Verification items for the finished model (mm, model axes). Coordinates: 2 decimals unless noted, no trailing zeros. Write each loop counter-clockwise with the first axis right and the second up, starting at its lowest first coordinate (ties: lowest second). Pieces come first, ordered by that corner, then holes. Notation, with made-up numbers: (53, -37.5) -> (61, -37.5) arc R15 cw to (61, -22.5) -> close; hole circle Ø7 at (14.5, -22.75). An arc over 180 degrees is marked (long way). Write item = value, one per line. Start each with the question number.
(1) Material ranges on probe 1 along X at (y, z) = (2.2, -17.96); probe 2 along X at (y, z) = (3.8, -18); probe 3 along Z at (x, y) = (3.5, 1.7), recorded low to high. Write a range as [from, to].
(2) Section check C-C (x = 9.5). Record the cut outline in (y, z), plus the area to 3 significant figures.
(3) Section check B-B (y = 3.15). Record the cut outline in (x, z), plus the area to 3 significant figures.
(4) Section check A-A (x = 24.56). Record the cut outline in (y, z).
(5) Gauge pin test, flat end, axial feed: pin 1 Ø0.6 at (x, y) = (13, 3.5) entering from +Z. Record the tip position at first contact, or that the pin passes through.
```python
from build123d import *

# Parameters (mm, degrees)
SKETCH1_W           = 27.1
SKETCH1_H           = 20.5
BOSS_EXTRUDE1_DEPTH = 4
SKETCH3_R           = 1.27
CUT_EXTRUDE1_DEPTH  = 35.214909031
SKETCH2_W           = 10.16
SKETCH2_H           = 1.27
SKETCH2_W_2         = 15.24
CUT_EXTRUDE2_DEPTH  = 0.508


with BuildPart() as part:
    # Sketch1 → Boss-Extrude1 (new body)
    with BuildSketch(Plane(origin=(0, 0, 0), x_dir=(1, 0, 0), z_dir=(0, 1, 0))):
        with Locations((13.55, 10.25)):
            Rectangle(SKETCH1_W, SKETCH1_H)
    extrude(amount=BOSS_EXTRUDE1_DEPTH)

    # Sketch3 → Cut-Extrude1 (cut, through all)
    with BuildSketch(Plane(origin=(0, 4, 0), x_dir=(1, 0, 0), z_dir=(0, 1, 0))):
        with Locations(Location((2.54, 17.96, 0), (0, 0, 270))):
            Circle(SKETCH3_R)
        with Locations(Location((2.54, 2.54, 0), (0, 0, 90))):
            Circle(SKETCH3_R)
        with Locations(Location((24.56, 2.54, 0), (0, 0, 270))):
            Circle(SKETCH3_R)
        with Locations(Location((24.56, 17.96, 0), (0, 0, 90))):
            Circle(SKETCH3_R)
    extrude(amount=-CUT_EXTRUDE1_DEPTH, mode=Mode.SUBTRACT)

    # Sketch2 → Cut-Extrude2 (cut)
    with BuildSketch(Plane(origin=(0, 4, 0), x_dir=(1, 0, 0), z_dir=(0, 1, 0))):
        with Locations((13.55, 18.595)):
            Rectangle(SKETCH2_W, SKETCH2_H)
        with Locations((13.55, 1.905)):
            Rectangle(SKETCH2_W_2, SKETCH2_H)
    extrude(amount=-CUT_EXTRUDE2_DEPTH, mode=Mode.SUBTRACT)


solid = part.part
```
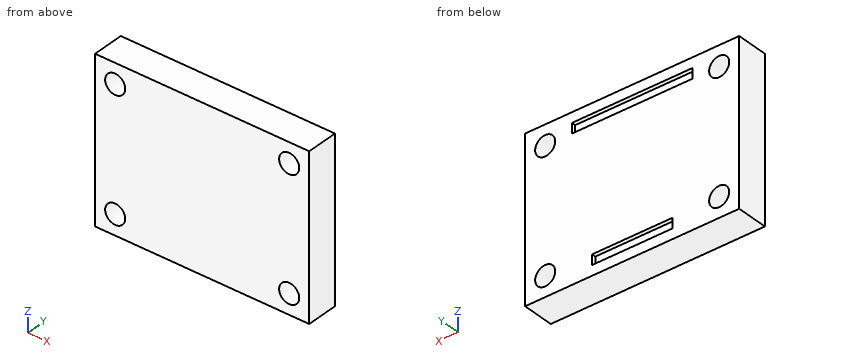
Response:
q1.probe_1 = [0, 1.27], [3.81, 23.29], [25.83, 27.1]
q1.probe_2 = [0, 1.27], [3.81, 8.47], [18.63, 23.29], [25.83, 27.1]
q1.probe_3 = [-20.5, -18.79], [-17.13, -3.37], [-1.71, 0]
q2.outline = (0, -20.5) -> (4, -20.5) -> (4, -19.23) -> (3.49, -19.23) -> (3.49, -17.96) -> (4, -17.96) -> (4, -2.54) -> (3.49, -2.54) -> (3.49, -1.27) -> (4, -1.27) -> (4, 0) -> (0, 0) -> close
q2.area = 80.7 mm2
q3.outline = (0, -20.5) -> (27.1, -20.5) -> (27.1, 0) -> (0, 0) -> close; hole circle Ø2.54 at (2.54, -17.96); hole circle Ø2.54 at (2.54, -2.54); hole circle Ø2.54 at (24.56, -17.96); hole circle Ø2.54 at (24.56, -2.54)
q3.area = 535 mm2
q4.outline = (0, -20.5) -> (4, -20.5) -> (4, -19.23) -> (0, -19.23) -> close; (0, -16.69) -> (4, -16.69) -> (4, -3.81) -> (0, -3.81) -> close; (0, -1.27) -> (4, -1.27) -> (4, 0) -> (0, 0) -> close
q5.pin_1 = 0
